The model under review builds one solid part; all positions refer to its coordinate system, in mm. A direction names the side the tool comes from. Give positions to 0.01 mm unless a question says otherwise; leave off trailing zeros. Order: outer loops, then holes, each group sorted by start corner. A loop starts at its lowest first (then second) coordinate and runs counter-clockwise, first axis right, second up.
```python
from build123d import *

# Parameters (mm, degrees)
SKETCH_1_R          = 10
SKETCH_1_R_2        = 4
EXTRUDE_1_DEPTH     = 10
EXTRUDE_2_DEPTH     = 5
SKETCH_4_R          = 2.75
CUT_EXTRUDE_6_DEPTH = 5
CUT_EXTRUDE_5_DEPTH = 5
EXTRUDE_3_DEPTH     = 10
CUT_EXTRUDE_8_DEPTH = 11
SKETCH_7_R          = 4.25
EXTRUDE_4_DEPTH     = 5


with BuildPart() as part:
    # 草图1 → 凸台-拉伸1 (new body)
    with BuildSketch(Plane.XY):
        Circle(SKETCH_1_R)
        Circle(SKETCH_1_R_2, mode=Mode.SUBTRACT)
    extrude(amount=EXTRUDE_1_DEPTH)

    # 草图2 → 凸台-拉伸2 (add)
    with BuildSketch(Plane.XY):
        with BuildLine():
            Line((2.8e-08, 10), (-21.5, 10))
            Line((-21.5, 10), (-21.5, -10))
            Line((-21.5, -10), (-1.9e-08, -10))
            ThreePointArc((-1.9e-08, -10), (-10, 2.4e-08), (2.8e-08, 10))
        make_face()
        with BuildLine():
            Line((21.5, 10), (2.8e-08, 10))
            ThreePointArc((2.8e-08, 10), (7.071067822, 7.071067802), (10, 0))
            ThreePointArc((10, 0), (7.071067805, -7.071067819), (-1.9e-08, -10))
            Line((-1.9e-08, -10), (21.5, -10))
            Line((21.5, -10), (21.5, 10))
        make_face()
    extrude(amount=EXTRUDE_2_DEPTH)

    # 草图4 → 切除-拉伸6 (cut)
    with BuildSketch(Plane.XY):
        with Locations((-16, 0)):
            Circle(SKETCH_4_R)
        with Locations((16, 0)):
            Circle(SKETCH_4_R)
    extrude(amount=CUT_EXTRUDE_6_DEPTH, mode=Mode.SUBTRACT)

    # 草图3 → 切除-拉伸5 (cut)
    with BuildSketch(Plane.XY):
        with BuildLine():
            ThreePointArc((-17.5625, -4.749588798), (-21, 0), (-17.5625, 4.749588798))
            Line((-17.5625, 4.749588798), (-3.125, 9.499177596))
            ThreePointArc((-3.125, 9.499177596), (-1.582438631, 9.874000607), (0, 10))
            Line((0, 10), (-21.5, 10))
            Line((-21.5, 10), (-21.5, -10))
            Line((-21.5, -10), (0, -10))
            ThreePointArc((0, -10), (-1.582438631, -9.874000607), (-3.125, -9.499177596))
            Line((-3.125, -9.499177596), (-17.5625, -4.749588798))
        make_face()
        with BuildLine():
            Line((21.5, 10), (0, 10))
            ThreePointArc((0, 10), (1.582438631, 9.874000607), (3.125, 9.499177596))
            Line((3.125, 9.499177596), (17.5625, 4.749588798))
            ThreePointArc((17.5625, 4.749588798), (20.050462937, 2.93150985), (21, 0))
            ThreePointArc((21, 0), (20.050462937, -2.93150985), (17.5625, -4.749588798))
            Line((17.5625, -4.749588798), (3.125, -9.499177596))
            ThreePointArc((3.125, -9.499177596), (1.582438631, -9.874000607), (0, -10))
            Line((0, -10), (21.5, -10))
            Line((21.5, -10), (21.5, 10))
        make_face()
        with BuildLine():
            Line((21.5, 10), (0, 10))
            ThreePointArc((0, 10), (1.582438631, 9.874000607), (3.125, 9.499177596))
            Line((3.125, 9.499177596), (17.5625, 4.749588798))
            ThreePointArc((17.5625, 4.749588798), (20.050462937, 2.93150985), (21, 0))
            ThreePointArc((21, 0), (20.050462937, -2.93150985), (17.5625, -4.749588798))
            Line((17.5625, -4.749588798), (3.125, -9.499177596))
            ThreePointArc((3.125, -9.499177596), (1.582438631, -9.874000607), (0, -10))
            Line((0, -10), (21.5, -10))
            Line((21.5, -10), (21.5, 10))
        make_face()
        with BuildLine():
            ThreePointArc((-17.5625, -4.749588798), (-21, 0), (-17.5625, 4.749588798))
            Line((-17.5625, 4.749588798), (-3.125, 9.499177596))
            ThreePointArc((-3.125, 9.499177596), (-1.582438631, 9.874000607), (0, 10))
            Line((0, 10), (-21.5, 10))
            Line((-21.5, 10), (-21.5, -10))
            Line((-21.5, -10), (0, -10))
            ThreePointArc((0, -10), (-1.582438631, -9.874000607), (-3.125, -9.499177596))
            Line((-3.125, -9.499177596), (-17.5625, -4.749588798))
        make_face()
    extrude(amount=CUT_EXTRUDE_5_DEPTH, mode=Mode.SUBTRACT)

    # 草图5 → 凸台-拉伸3 (add)
    with BuildSketch(Plane.XY):
        with BuildLine():
            Line((-8, -6), (-8, -12))
            Line((-8, -12), (8, -12))
            Line((8, -12), (8, -6))
            ThreePointArc((8, -6), (0, -10), (-8, -6))
        make_face()
    extrude(amount=EXTRUDE_3_DEPTH)

    # 草图6 → 切除-拉伸8 (cut, through all)
    with BuildSketch(Plane.XY):
        with BuildLine():
            Line((-0.6, -12), (0.6, -12))
            Line((0.6, -12), (0.6, -3.954743987))
            ThreePointArc((0.6, -3.954743987), (0, -4), (-0.6, -3.954743987))
            Line((-0.6, -3.954743987), (-0.6, -12))
        make_face()
    extrude(amount=CUT_EXTRUDE_8_DEPTH, mode=Mode.SUBTRACT)

    # 草图7 → 凸台-拉伸4 (add)
    with BuildSketch(Plane.XY.offset(5)):
        with BuildLine():
            Line((-17.5625, -4.749588798), (-8, -7.89542034))
            Line((-8, -7.89542034), (-8, -6))
            ThreePointArc((-8, -6), (-9.539262696, 3.000411174), (-3.125, 9.499177596))
            Line((-3.125, 9.499177596), (-17.5625, 4.749588798))
            ThreePointArc((-17.5625, 4.749588798), (-21, 0), (-17.5625, -4.749588798))
        make_face()
        with Locations((-16, 0)):
            Circle(SKETCH_7_R, mode=Mode.SUBTRACT)
        with BuildLine():
            Line((8, -6), (8, -7.89542034))
            Line((8, -7.89542034), (17.5625, -4.749588798))
            ThreePointArc((17.5625, -4.749588798), (21, 0), (17.5625, 4.749588798))
            Line((17.5625, 4.749588798), (3.125, 9.499177596))
            ThreePointArc((3.125, 9.499177596), (9.539262696, 3.000411174), (8, -6))
        make_face()
        with Locations((16, 0)):
            Circle(SKETCH_7_R, mode=Mode.SUBTRACT)
    extrude(amount=EXTRUDE_4_DEPTH)


solid = part.part
```
Item 1: Take a section at B-B (z = 2.5). Give the number of separate pieces and of enclosed holes in the cut face, and give its area (3 significant figures).
Values found:
separate pieces: 1
enclosed holes: 2
area: 521 mm2
Item 2: For line 1 (X direction, y = -9.5, z = 2.5); line 2 (X direction, y = 1, z = 3.75); line 3 (X direction, y = -1, z = 8.5), list the stretches that pass through material, from the lowest coordinate up.
Values found:
line 1: x = -8 to -0.6, 0.6 to 8
line 2: x = -20.9 to -18.56, -13.44 to -3.87, 3.87 to 13.44, 18.56 to 20.9
line 3: x = -20.9 to -20.13, -11.87 to -3.87, 3.87 to 11.87, 20.13 to 20.9
Item 3: Take a section at C-C (y = 0.75). Give the boundary of the cut face in (x, z), and give its area (3 significant figures).
Values found:
outline: (-20.94, 0) - (-18.65, 0) - (-18.65, 5) - (-20.18, 5) - (-20.18, 10) - (-20.94, 10) - close; (-13.35, 0) - (-3.93, 0) - (-3.93, 10) - (-11.82, 10) - (-11.82, 5) - (-13.35, 5) - close; (3.93, 0) - (13.35, 0) - (13.35, 5) - (11.82, 5) - (11.82, 10) - (3.93, 10) - close; (18.65, 0) - (20.94, 0) - (20.94, 10) - (20.18, 10) - (20.18, 5) - (18.65, 5) - close
area: 204 mm2
Item 4: Draft analysis for pull direction X (two halves, no side actions). For faces 1 (the flat face through (-4, -12, 5)), 2 (the flat face through (10.24, 7.16, 4.93)), 3 (the flat face through (-0.6, -8, 5)), state which applies: released by +X, released by -X, zero draft, split by the parting line, or undercut.
Values found:
face 1: zero draft
face 2: released by +X
face 3: undercut
Item 5: For faces 4 (the flat face through (-8, -10, 5)), 5 (the flat face through (16, -3, 5)), 6 (the flat face through (0.6, -8, 5)), list the 3-axis set-ups (+Z, -Z, +X, -X, +Y, -Y) from which the entire face can be reached by the end or side of a thin tool; tool diameter is ignored.
Values found:
face 4: +Z, -Z, -X, -Y
face 5: +Z
face 6: +Z, -Z, -Y
Item 6: Take a section at D-D (x = -16). Give the boundary of the cut face in (y, z).
Values found:
outline: (-5.26, 0) - (-2.75, 0) - (-2.75, 5) - (-4.25, 5) - (-4.25, 10) - (-5.26, 10) - close; (2.75, 0) - (5.26, 0) - (5.26, 10) - (4.25, 10) - (4.25, 5) - (2.75, 5) - close
Item 7: Clearance check with flat-ended pins moving along their axes: pin 1 Ø3 at (y, z) = (4, 3.5) entering from +X; pin 2 Ø7.5 at (x, y) = (-16, 0) entering from +Z; pin 3 Ø4.5 at (y, z) = (-10.5, 6) entering from -X. State where each tip first meets the part, or that it passes through.
Values found:
pin 1: stops at x = 20.33
pin 2: stops at z = 5
pin 3: stops at x = -8
Item 8: Take a section at A-A (y = -8.75). Give the boundary of the cut face in (x, z), and give its area (3 significant figures).
Values found:
outline: (-8, 0) - (-0.6, 0) - (-0.6, 10) - (-8, 10) - close; (0.6, 0) - (8, 0) - (8, 10) - (0.6, 10) - close
area: 148 mm2
